The model under review builds one solid part; all positions refer to its coordinate system, in mm. Face numbers are marked on the shaded views. Round coordinates to 2 decimals unless told otherwise and drop trailing zeros. Order: outer loops, then holes, each group sorted by start corner. A loop starts at its lowest first (then second) coordinate and runs counter-clockwise, first axis right, second up. Notation, with made-up numbers: M 4.25,83.5 L 25.25,83.5 A35 cw 25.25,115.5 Z; hole C -8,75 d2. An arc over 180 degrees is marked long. Use a Markdown table: item, result. Add a question column.
1. Consider section C-C on z = -94. State the section outline as (x, y) points.
2. To check wall thickness, follow probe 1 along Y at (x, z) = (0, 5.75); probe 2 along Y at (x, z) = (0, -77); probe 3 along Z at (x, y) = (7, -15). State the ranges of each line that lie inside material, in increasing order.
3. Consider section A-A on y = 0. State the section outline as (x, z) points, then the cut area to 3 significant figures.
4. The part is to be moulded in two halves that separate along X. For the marked faces 1, 2 and 3, say which applies: +X half, -X half, draft (parallel to the pull), parting line (faces both ways), or undercut.
5. Insertion check: P1, Ø1.5, axis at x = 31, y = 29.5, coming from the -Z side; P2, Ø4, axis at x = -73, y = -42, coming from the -Z side; P3, Ø25, axis at x = 0, y = 0, coming from the -Z side. Each pin has a flat end and moves straight along its axis. Give the tip position at first contact, or say it passes through.
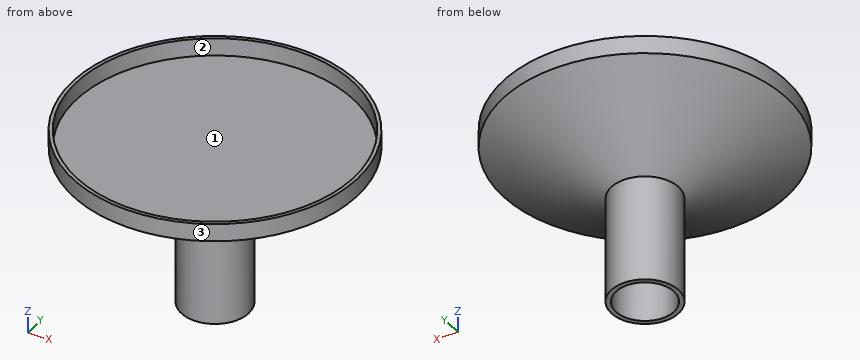
from build123d import *

# Parameters (mm, degrees)
SKETCH1_R           = 101.6
BOSS_EXTRUDE1_DEPTH = 12.7
SKETCH4_R           = 99.06
CUT_EXTRUDE1_DEPTH  = 38.1
SKETCH6_R           = 24.13
SKETCH6_R_2         = 20.828
BOSS_EXTRUDE2_DEPTH = 76.2


with BuildPart() as part:
    # Sketch1 → Boss-Extrude1 (new body)
    with BuildSketch(Plane.XY):
        Circle(SKETCH1_R)
    extrude(amount=BOSS_EXTRUDE1_DEPTH)

    # Sketch4 → Cut-Extrude1 (cut)
    with BuildSketch(Plane.XY.offset(12.7)):
        Circle(SKETCH4_R)
    extrude(amount=-CUT_EXTRUDE1_DEPTH, mode=Mode.SUBTRACT)



with BuildPart() as body_2:
    # Sketch6 → Boss-Extrude2 (new body)
    with BuildSketch(Plane(origin=(0, 0, -38.1), x_dir=(-1, 0, 0), z_dir=(0, 0, -1))):
        with Locations(Location((0, 0, 0), (0, 0, 180))):
            Circle(SKETCH6_R)
        with Locations(Location((0, 0, 0), (0, 0, 180))):
            Circle(SKETCH6_R_2, mode=Mode.SUBTRACT)
    extrude(amount=BOSS_EXTRUDE2_DEPTH)


with BuildPart() as part_1:
    add(part.part)

    add(body_2.part)  # Loft2 merges body 2
    # Loft2: read off the stored shape, not the designer's step
    # Loft2 outline → Loft2 (revolve)
    with BuildSketch(Plane.XZ):
        Polygon((101.6, 0), (0, 0), (0, -38.1), (24.13, -38.1), align=None)
    revolve(axis=Axis((0, 0, 0), (0, 0, 1)))


solid = part_1.part
Answer block:
| question | item | result |
|---|---|---|
| 1 | outline | C 0,0 d48.26; hole C 0,0 d41.66 |
| 2 | probe 1 | -101.6 to -99.06, 99.06 to 101.6 |
| 2 | probe 2 | -24.13 to -20.83, 20.83 to 24.13 |
| 2 | probe 3 | -38.1 to 0 |
| 3 | outline | M -101.6,0 L -24.13,-38.1 L -24.13,-114.3 L -20.83,-114.3 L -20.83,-38.1 L 20.83,-38.1 L 20.83,-114.3 L 24.13,-114.3 L 24.13,-38.1 L 101.6,0 L 101.6,12.7 L 99.06,12.7 L 99.06,0 L -99.06,0 L -99.06,12.7 L -101.6,12.7 Z |
| 3 | area | 5,360 mm^2 |
| 4 | face 1 | undercut |
| 4 | face 2 | undercut |
| 4 | face 3 | parting line |
| 5 | P1 | z = -29.29 |
| 5 | P2 | z = -9.53 |
| 5 | P3 | z = -38.1 |
